Check sheet for the drawn part. Datum: minimum x, y, z corner. Units: mm. Give positions to 0.01 mm unless a question says otherwise; leave off trailing zeros. Write each loop counter-clockwise with the first axis right and the second up, starting at its lowest first coordinate (ties: lowest second). Pieces come first, ordered by that corner, then holes.
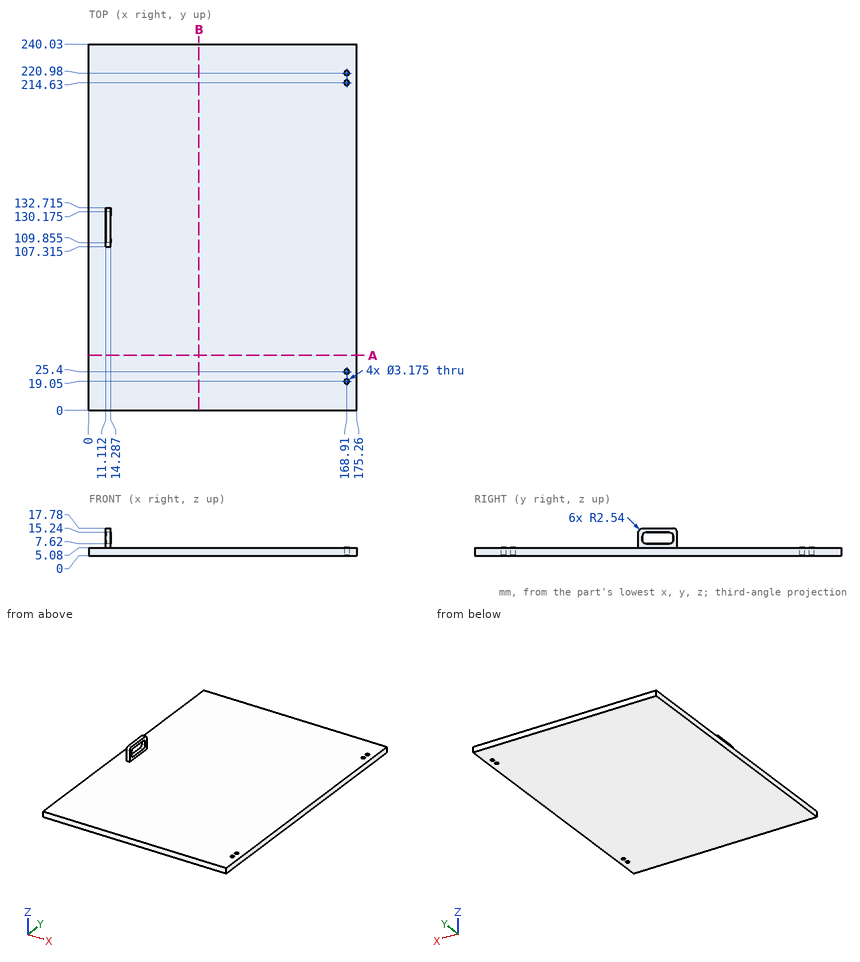
1) Sectioned sample at B-B on x = 72. Record the boundary of the cut face in (y, z).
2) Sectioned sample at A-A on y = 36. Record the boundary of the cut face in (x, z).
3) Gauge pin test, flat ends, axial feed: pin 1 (0.8 mm diameter, centred on x = 12, z = 12, fed in from -Y) (1 decimal); pin 2 (4 mm diameter, centred on x = 168.91, y = 214.63, fed in from -Z); pin 3 (1.3 mm diameter, centred on x = 13, z = 12, fed in from +Y) (1 decimal); pin 4 (4 mm diameter, centred on x = 37.5, y = 111.5, fed in from +Z). Record the tip position at first contact, or that the pin passes through.
4) Scan lines: L1, parallel to Y at x = 168.91, z = 2.55; L2, parallel to X at y = 214.63, z = 1.85; L3, parallel to Z at x = 148.5, y = 105. Record each from-to range of solid material in increasing order.
Answers below:
1. outline: (0, 0) - (240.03, 0) - (240.03, 5.08) - (0, 5.08) - close
2. outline: (0, 0) - (175.26, 0) - (175.26, 5.08) - (0, 5.08) - close
3. pin 1: stops at y = 107.3
3. pin 2: stops at z = 0
3. pin 3: stops at y = 132.7
3. pin 4: stops at z = 5.08
4. L1: y = 0 to 17.46, 20.64 to 23.81, 26.99 to 213.04, 216.22 to 219.39, 222.57 to 240.03
4. L2: x = 0 to 167.32, 170.5 to 175.26
4. L3: z = 0 to 5.08
